Build history of the part. All positions in model axes, mm. Give positions to 0.01 mm unless a question says otherwise; leave off trailing zeros. Write each loop counter-clockwise with the first axis right and the second up, starting at its lowest first coordinate (ties: lowest second). Pieces come first, ordered by that corner, then holes. Notation, with made-up numbers: (65.25, 13.25) -> (87.25, 13.25) arc R33 cw to (87.25, 46.25) -> close; hole circle Ø1 at (41, -24.75). An arc over 180 degrees is marked (long way). Put each result on its own line as item: value.
from build123d import *
from OCP.BRepFilletAPI import BRepFilletAPI_MakeChamfer

# Parameters (mm, degrees)
SKETCH_1_W                          = 2.54
SKETCH_1_H                          = 2.54
EXTRUDE_1_DEPTH                     = 8.51
SKETCH_4_W                          = 0.7
SKETCH_4_H                          = 0.7
CUT_EXTRUDE_1_DEPTH                 = 8.21
CHAMFER_3_SIZE                      = 0.4
SKETCH_2_W                          = 0.5
SKETCH_2_H                          = 0.5
EXTRUDE_2_DEPTH                     = 3.15
CHAMFER_2_SIZE                      = 0.5
CHAMFER_2_SIZE2                     = 0.106278281
PATTERN_LINEAR_1_COUNT              = 2
PATTERN_LINEAR_1_PITCH              = 2.54
PATTERN_LINEAR_1_COUNT_DIR2         = 2
PATTERN_LINEAR_1_PITCH_DIR2         = 2.54
CHAMFER_3_OF_PATTERN_LINEAR_1_SIZE  = 0.4
CHAMFER_2_OF_PATTERN_LINEAR_1_SIZE  = 0.5
CHAMFER_2_OF_PATTERN_LINEAR_1_SIZE2 = 0.106278281


with BuildPart() as part:
    # Эскиз1 → Бобышка-Вытянуть1 (new body)
    with BuildSketch(Plane(origin=(0, 0, 0), x_dir=(-1, 0, 0), z_dir=(0, 1, 0))):
        Rectangle(SKETCH_1_W, SKETCH_1_H)
    extrude_1 = extrude(amount=EXTRUDE_1_DEPTH)

    # Эскиз4 → Вырез-Вытянуть1 (cut)
    with BuildSketch(Plane(origin=(0, 8.51, 0), x_dir=(1, 0, 0), z_dir=(0, 1, 0))):
        Rectangle(SKETCH_4_W, SKETCH_4_H)
    cut_extrude_1 = extrude(amount=-CUT_EXTRUDE_1_DEPTH, mode=Mode.SUBTRACT)

    # Фаска3
    chamfer_3_edges = [part.edges().sort_by_distance(p)[0] for p in [
        (-0.35, 8.51, 0),
        (0, 8.51, 0.35),
        (0.35, 8.51, 0),
        (0, 8.51, -0.35),
    ]]
    chamfer(chamfer_3_edges, length=CHAMFER_3_SIZE)

    # Эскиз2 → Бобышка-Вытянуть2 (add)
    with BuildSketch(Plane(origin=(0, 0, 0), x_dir=(-1, 0, 0), z_dir=(0, 1, 0))):
        Rectangle(SKETCH_2_W, SKETCH_2_H)
    extrude_2 = extrude(amount=-EXTRUDE_2_DEPTH)

    # Фаска2: one chamfer whose edges measure the first distance from different faces: ONE call of the kernel's chamfer builder (chamfer() names one face for all edges)
    chamfer_2_edges_1 = [part.edges().sort_by_distance(p)[0] for p in [
        (-0.25, -3.15, 0),
    ]]
    chamfer_2_side_1 = [part.faces().sort_by_distance(p)[0] for p in [
        (-0.25, -1.575, 0),
    ]]
    chamfer_2_edges_2 = [part.edges().sort_by_distance(p)[0] for p in [
        (0.25, -3.15, 0),
    ]]
    chamfer_2_side_2 = [part.faces().sort_by_distance(p)[0] for p in [
        (0.25, -1.575, 0),
    ]]
    chamfer_2 = BRepFilletAPI_MakeChamfer(part.part.solid().wrapped)
    for e in chamfer_2_edges_1:
        chamfer_2.Add(CHAMFER_2_SIZE, CHAMFER_2_SIZE2, e.wrapped, chamfer_2_side_1[0].wrapped)  # the first distance lies on this face
    for e in chamfer_2_edges_2:
        chamfer_2.Add(CHAMFER_2_SIZE, CHAMFER_2_SIZE2, e.wrapped, chamfer_2_side_2[0].wrapped)  # the first distance lies on this face
    add(Compound.cast(chamfer_2.Shape()), mode=Mode.REPLACE)

    # Линейный массив1: Бобышка-Вытянуть1, Вырез-Вытянуть1, Extrude 2 2 × 2
    with Locations(*[(-j * PATTERN_LINEAR_1_PITCH_DIR2, 0, -i * PATTERN_LINEAR_1_PITCH) for i in range(PATTERN_LINEAR_1_COUNT) for j in range(PATTERN_LINEAR_1_COUNT_DIR2) if (i, j) != (0, 0)]):
        add(extrude_1)
        add(cut_extrude_1, mode=Mode.SUBTRACT)
        add(extrude_2)

    # Фаска3 of Линейный массив1
    chamfer_3_of_pattern_linear_1_edges = [part.edges().sort_by_distance(p)[0] for p in [
        (-2.89, 8.51, 0),
        (-2.54, 8.51, 0.35),
        (-2.19, 8.51, 0),
        (-2.54, 8.51, -0.35),
        (-0.35, 8.51, -2.54),
        (0, 8.51, -2.19),
        (0.35, 8.51, -2.54),
        (0, 8.51, -2.89),
        (-2.89, 8.51, -2.54),
        (-2.54, 8.51, -2.19),
        (-2.19, 8.51, -2.54),
        (-2.54, 8.51, -2.89),
    ]]
    chamfer(chamfer_3_of_pattern_linear_1_edges, length=CHAMFER_3_OF_PATTERN_LINEAR_1_SIZE)

    # Фаска2 of Линейный массив1: one chamfer whose edges measure the first distance from different faces: ONE call of the kernel's chamfer builder (chamfer() names one face for all edges)
    chamfer_2_of_pattern_linear_1_edges_1 = [part.edges().sort_by_distance(p)[0] for p in [
        (-2.79, -3.15, 0),
    ]]
    chamfer_2_of_pattern_linear_1_side_1 = [part.faces().sort_by_distance(p)[0] for p in [
        (-2.79, -1.575, 0),
    ]]
    chamfer_2_of_pattern_linear_1_edges_2 = [part.edges().sort_by_distance(p)[0] for p in [
        (-2.29, -3.15, 0),
    ]]
    chamfer_2_of_pattern_linear_1_side_2 = [part.faces().sort_by_distance(p)[0] for p in [
        (-2.29, -1.575, 0),
    ]]
    chamfer_2_of_pattern_linear_1_edges_3 = [part.edges().sort_by_distance(p)[0] for p in [
        (-0.25, -3.15, -2.54),
    ]]
    chamfer_2_of_pattern_linear_1_side_3 = [part.faces().sort_by_distance(p)[0] for p in [
        (-0.25, -1.575, -2.54),
    ]]
    chamfer_2_of_pattern_linear_1_edges_4 = [part.edges().sort_by_distance(p)[0] for p in [
        (0.25, -3.15, -2.54),
    ]]
    chamfer_2_of_pattern_linear_1_side_4 = [part.faces().sort_by_distance(p)[0] for p in [
        (0.25, -1.575, -2.54),
    ]]
    chamfer_2_of_pattern_linear_1_edges_5 = [part.edges().sort_by_distance(p)[0] for p in [
        (-2.79, -3.15, -2.54),
    ]]
    chamfer_2_of_pattern_linear_1_side_5 = [part.faces().sort_by_distance(p)[0] for p in [
        (-2.79, -1.575, -2.54),
    ]]
    chamfer_2_of_pattern_linear_1_edges_6 = [part.edges().sort_by_distance(p)[0] for p in [
        (-2.29, -3.15, -2.54),
    ]]
    chamfer_2_of_pattern_linear_1_side_6 = [part.faces().sort_by_distance(p)[0] for p in [
        (-2.29, -1.575, -2.54),
    ]]
    chamfer_2_of_pattern_linear_1 = BRepFilletAPI_MakeChamfer(part.part.solid().wrapped)
    for e in chamfer_2_of_pattern_linear_1_edges_1:
        chamfer_2_of_pattern_linear_1.Add(CHAMFER_2_OF_PATTERN_LINEAR_1_SIZE, CHAMFER_2_OF_PATTERN_LINEAR_1_SIZE2, e.wrapped, chamfer_2_of_pattern_linear_1_side_1[0].wrapped)  # the first distance lies on this face
    for e in chamfer_2_of_pattern_linear_1_edges_2:
        chamfer_2_of_pattern_linear_1.Add(CHAMFER_2_OF_PATTERN_LINEAR_1_SIZE, CHAMFER_2_OF_PATTERN_LINEAR_1_SIZE2, e.wrapped, chamfer_2_of_pattern_linear_1_side_2[0].wrapped)  # the first distance lies on this face
    for e in chamfer_2_of_pattern_linear_1_edges_3:
        chamfer_2_of_pattern_linear_1.Add(CHAMFER_2_OF_PATTERN_LINEAR_1_SIZE, CHAMFER_2_OF_PATTERN_LINEAR_1_SIZE2, e.wrapped, chamfer_2_of_pattern_linear_1_side_3[0].wrapped)  # the first distance lies on this face
    for e in chamfer_2_of_pattern_linear_1_edges_4:
        chamfer_2_of_pattern_linear_1.Add(CHAMFER_2_OF_PATTERN_LINEAR_1_SIZE, CHAMFER_2_OF_PATTERN_LINEAR_1_SIZE2, e.wrapped, chamfer_2_of_pattern_linear_1_side_4[0].wrapped)  # the first distance lies on this face
    for e in chamfer_2_of_pattern_linear_1_edges_5:
        chamfer_2_of_pattern_linear_1.Add(CHAMFER_2_OF_PATTERN_LINEAR_1_SIZE, CHAMFER_2_OF_PATTERN_LINEAR_1_SIZE2, e.wrapped, chamfer_2_of_pattern_linear_1_side_5[0].wrapped)  # the first distance lies on this face
    for e in chamfer_2_of_pattern_linear_1_edges_6:
        chamfer_2_of_pattern_linear_1.Add(CHAMFER_2_OF_PATTERN_LINEAR_1_SIZE, CHAMFER_2_OF_PATTERN_LINEAR_1_SIZE2, e.wrapped, chamfer_2_of_pattern_linear_1_side_6[0].wrapped)  # the first distance lies on this face
    add(Compound.cast(chamfer_2_of_pattern_linear_1.Shape()), mode=Mode.REPLACE)


solid = part.part
1) Slice it at D-D (z = -3.15). Write the cut outline in (x, y).
Filled sheet:
outline: (-3.81, 0) -> (1.27, 0) -> (1.27, 8.51) -> (0.75, 8.51) -> (0.61, 8.37) -> (-0.61, 8.37) -> (-0.75, 8.51) -> (-1.79, 8.51) -> (-1.93, 8.37) -> (-3.15, 8.37) -> (-3.29, 8.51) -> (-3.81, 8.51) -> close
2) Slice it at B-B (y = 4.25). Write the cut outline in (x, z), plus the area to 3 significant figures.
Filled sheet:
outline: (-3.81, -3.81) -> (1.27, -3.81) -> (1.27, 1.27) -> (-3.81, 1.27) -> close; hole (-2.89, -2.89) -> (-2.19, -2.89) -> (-2.19, -2.19) -> (-2.89, -2.19) -> close; hole (-2.89, -0.35) -> (-2.19, -0.35) -> (-2.19, 0.35) -> (-2.89, 0.35) -> close; hole (-0.35, -2.89) -> (0.35, -2.89) -> (0.35, -2.19) -> (-0.35, -2.19) -> close; hole (-0.35, -0.35) -> (0.35, -0.35) -> (0.35, 0.35) -> (-0.35, 0.35) -> close
area: 23.8 mm2
3) Slice it at A-A (y = -2). Write the cut outline in (x, z), plus the area to 3 significant figures.
Filled sheet:
outline: (-2.79, -2.79) -> (-2.29, -2.79) -> (-2.29, -2.29) -> (-2.79, -2.29) -> close; (-2.79, -0.25) -> (-2.29, -0.25) -> (-2.29, 0.25) -> (-2.79, 0.25) -> close; (-0.25, -2.79) -> (0.25, -2.79) -> (0.25, -2.29) -> (-0.25, -2.29) -> close; (-0.25, -0.25) -> (0.25, -0.25) -> (0.25, 0.25) -> (-0.25, 0.25) -> close
area: 1.00 mm2
4) Pin check, flat tips, straight feed: pin 1 (0.6 mm diameter, centred on y = -1, z = 0, fed in from +X); pin 2 (0.6 mm diameter, centred on x = -2.5, y = -2, fed in from -Z). Stop position of each tip, or through.
Filled sheet:
pin 1: x = 0.25
pin 2: z = -2.79
5) Wall check: L1, parallel to Z at x = -0.2, y = 4.75. Give the ranges that are in metal, low to high.
Filled sheet:
L1: -3.81 to -2.89, -2.19 to -0.35, 0.35 to 1.27
6) Slice it at C-C (x = -3.15). Write the cut outline in (y, z).
Filled sheet:
outline: (0, -3.81) -> (8.51, -3.81) -> (8.51, -3.29) -> (8.37, -3.15) -> (8.37, -1.93) -> (8.51, -1.79) -> (8.51, -0.75) -> (8.37, -0.61) -> (8.37, 0.61) -> (8.51, 0.75) -> (8.51, 1.27) -> (0, 1.27) -> close
